Input: part model. Units: mm. Frame: model coordinates. Face numbers are marked on the shaded views. A direction names the side the tool comes from. Round coordinates to 2 decimals unless told otherwise and drop trailing zeros. Loops run counter-clockwise (first coordinate to the right, second up) from the corner with the lowest first, then second, coordinate; pieces in that order, holes last. Notation, with made-up numbers: (89, 9.5) -> (117, 9.5) arc R30 cw to (117, 45.5) -> close; hole circle Ø1 at (-35.5, 84). An arc over 180 degrees is marked (long way). Answer as a JSON object with one key per item and string values. Group by question number.
Item 1: Section query B-B on z = -17. Return loops of the section in (x, y), and give its area (3 significant figures).
Item 2: Section query C-C on y = 70. Return loops of the section in (x, z), and give its area (4 significant figures).
Item 3: Section query A-A on x = -8.75. Return loops of the section in (y, z).
Item 4: Material intervals for line 1 (Z direction, x = 10.5, y = 70); line 2 (Y direction, x = 9, z = -35.8); line 3 (X direction, y = 101, z = -41), sorted ascending. Write a range as [from, to].
Item 5: Pin query (flat end, axial travel): pin 1 (2.5 mm diameter, centred on y = 70, z = -17, fed in from +X); pin 2 (4 mm diameter, centred on y = 46, z = -35.8, fed in from +X); pin 3 (1.5 mm diameter, centred on x = -8.5, z = -14, fed in from -Y); pin 4 (10 mm diameter, centred on x = -7, y = 52, fed in from +Z). Return the tip coordinate at first contact, or that it passes through.
Item 6: Section query D-D on z = -28. Return loops of the section in (x, y).
Item 7: Set-up query: the marked faces 1, 2, 3, 4 and 5. Return all of +Z, -Z, +X, -X, +Y, -Y with unobstructed straight access to the full face (end or side cutting, diameter ignored); none if empty.
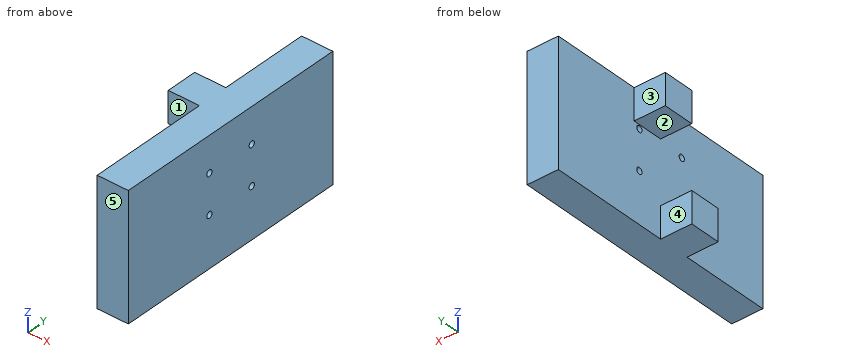
from build123d import *

# Parameters (mm, degrees)
CROQUIS1_W              = 60
CROQUIS1_H              = 116
SALIENTE_EXTRUIR1_DEPTH = 15
CROQUIS2_W              = 15
CROQUIS2_H              = 15
SALIENTE_EXTRUIR2_DEPTH = 15
CROQUIS3_R              = 1.5
CORTAR_EXTRUIR1_DEPTH   = 135


with BuildPart() as part:
    # Croquis1 → Saliente-Extruir1 (new body)
    with BuildSketch(Plane(origin=(0, 0, 0), x_dir=(0, 0, -1), z_dir=(1, 0, 0))):
        with Locations((30, 58)):
            Rectangle(CROQUIS1_W, CROQUIS1_H)
    extrude(amount=SALIENTE_EXTRUIR1_DEPTH)

    # Croquis2 → Saliente-Extruir2 (add)
    with BuildSketch(Plane.ZY):
        with Locations((-52.5, 50.5)):
            Rectangle(CROQUIS2_W, CROQUIS2_H)
        with Locations((-7.5, 65.5)):
            Rectangle(CROQUIS2_W, CROQUIS2_H)
    extrude(amount=SALIENTE_EXTRUIR2_DEPTH)

    # Croquis3 → Cortar-Extruir1 (cut, through all)
    with BuildSketch(Plane(origin=(15, 0, 0), x_dir=(0, 0, -1), z_dir=(1, 0, 0))):
        with Locations((17, 70)):
            Circle(CROQUIS3_R)
        with Locations((17, 46)):
            Circle(CROQUIS3_R)
        with Locations((35.8, 70)):
            Circle(CROQUIS3_R)
        with Locations((35.8, 46)):
            Circle(CROQUIS3_R)
    extrude(amount=-CORTAR_EXTRUIR1_DEPTH, mode=Mode.SUBTRACT)


solid = part.part
Solved:
{
 "1": {"outline": "(0, 0) -> (15, 0) -> (15, 44.5) -> (0, 44.5) -> close; (0, 47.5) -> (15, 47.5) -> (15, 68.5) -> (0, 68.5) -> close; (0, 71.5) -> (15, 71.5) -> (15, 116) -> (0, 116) -> close", "area": "1,650 mm²"},
 "2": {"outline": "(-15, -15) -> (0, -15) -> (0, -15.5) -> (15, -15.5) -> (15, 0) -> (-15, 0) -> close; (0, -60) -> (15, -60) -> (15, -37.3) -> (0, -37.3) -> close; (0, -34.3) -> (15, -34.3) -> (15, -18.5) -> (0, -18.5) -> close", "area": "1,035 mm²"},
 "3": {"outline": "(43, -60) -> (58, -60) -> (58, -45) -> (43, -45) -> close; (58, -15) -> (73, -15) -> (73, 0) -> (58, 0) -> close"},
 "4": {"line 1": "[-60, -37.3], [-34.3, -18.5], [-15.5, 0]", "line 2": "[0, 44.5], [47.5, 68.5], [71.5, 116]", "line 3": "[0, 15]"},
 "5": {"pin 1": "through", "pin 2": "x = 15", "pin 3": "y = 58", "pin 4": "z = -45"},
 "6": {"outline": "(0, 0) -> (15, 0) -> (15, 116) -> (0, 116) -> close"},
 "7": {"face 1": "+Z, -X, -Y", "face 2": "-Z, -X, +Y, -Y", "face 3": "+Z, -Z, -X, +Y", "face 4": "-Z, -X, +Y", "face 5": "+Z, -Z, +X, -X, -Y"}
}
